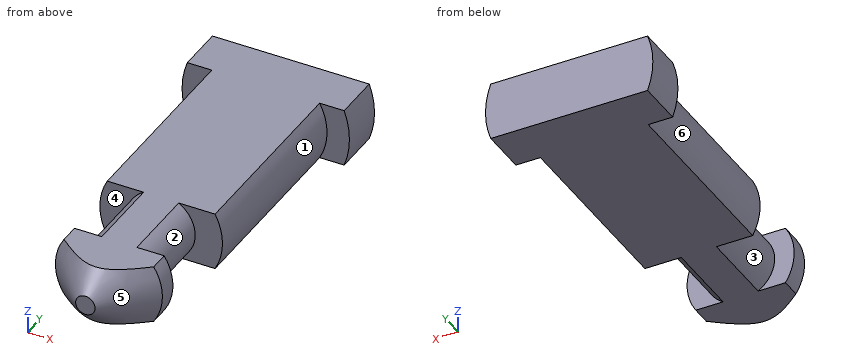
from build123d import *

# Parameters (mm, degrees)
F2_W     = 15
F2_H     = 3
F3_DEPTH = 25


with BuildPart() as f1:
    # F0 (on Top) → F1 (revolve)
    with BuildSketch(Plane.XY):
        Polygon((0, 19.65), (0, 0), (0.5, 0), (2.75, 2.25), (2.75, 3.25), (1.75, 3.25), (1.75, 7.25), (3.15, 7.25), (3.15, 17.25), (4.3, 17.25), (4.3, 19.65), align=None)
    revolve(axis=Axis((0, 9.825, 0), (0, 1, 0)))


with BuildPart() as f3:
    # F2 (on face) → F3 (new body)
    with BuildSketch(Plane(origin=(0, 19.65, 0), x_dir=(-1, 0, 0), z_dir=(0, 1, 0))):
        Rectangle(F2_W, F2_H)
    extrude(amount=-F3_DEPTH)

    # F4: intersect F1
    add(f1.part, mode=Mode.INTERSECT)


solid = f3.part
Verification items for the finished model (mm, model axes). Face numbers are marked on the shaded views. A direction names the side the tool comes from. Give positions to 0.01 mm unless a question says otherwise; leave off trailing zeros. Write each loop counter-clockwise with the first axis right and the second up, starting at its lowest first coordinate (ties: lowest second). Pieces come first, ordered by that corner, then holes. Notation, with made-up numbers: (5, 23.5) - (35, 23.5) arc R31 ccw to (35, 53.5) - close; hole circle Ø5 at (80, 70). An arc over 180 degrees is marked (long way). Answer as CSV lines item,"result". Start each with the question number.
1. Thickness scan on line 1 (Y direction, x = 3.25, z = -1.25); line 2 (Y direction, x = 2.25, z = 0.8); line 3 (Y direction, x = 2.75, z = -0.9). Record the ranges inside material, lowest first.
2. Sectioned sample at D-D (y = 11.5). Record the boundary of the cut face in (x, z).
3. Draft check along Y on the marked faces 4, 5 and 6. Enter one of: pulls with the +Y half, pulls with the -Y half, needs draft (parallel to the pull), parting line crosses it, or undercut.
4. Depth check by flat-ended pin: pin 1 (0.5 mm diameter, centred on x = 3.5, z = 0, fed in from -Y); pin 2 (0.8 mm diameter, centred on x = -3.5, z = 0, fed in from -Y); pin 3 (1.8 mm diameter, centred on x = 2.5, z = -0.5, fed in from -Y). Enter the tip coordinate at first touch or a pass-through.
5. Set-up check for the marked faces 1, 2 and 3: record each of +Z, -Z, +X, -X, +Y, -Y from which the full face is reachable in a straight line by a thin tool's end or side.
6. Sectioned sample at A-A (z = 0). Record the boundary of the cut face in (x, y).
7. Sectioned sample at B-B (x = 0). Record the boundary of the cut face in (y, z).
8. Sectioned sample at C-C (y = 6.75). Record the boundary of the cut face in (x, z), then the cut area to 3 significant figures.
Derived:
1,line 1,"17.25 to 19.65"
1,line 2,"1.89 to 3.25, 7.25 to 19.65"
1,line 3,"7.25 to 19.65"
2,outline,"(-2.77, -1.5) - (2.77, -1.5) arc R3.15 ccw to (2.77, 1.5) - (-2.77, 1.5) arc R3.15 ccw to start"
3,face 4,"undercut"
3,face 5,"pulls with the -Y half"
3,face 6,"needs draft"
4,pin 1,"y = 17.25"
4,pin 2,"y = 7.25"
4,pin 3,"y = 1.15"
5,face 1,"+X, -Y"
5,face 2,"+X"
5,face 3,"-X"
6,outline,"(-4.3, 17.25) - (-3.15, 17.25) - (-3.15, 7.25) - (-1.75, 7.25) - (-1.75, 3.25) - (-2.75, 3.25) - (-2.75, 2.25) - (-0.5, 0) - (0.5, 0) - (2.75, 2.25) - (2.75, 3.25) - (1.75, 3.25) - (1.75, 7.25) - (3.15, 7.25) - (3.15, 17.25) - (4.3, 17.25) - (4.3, 19.65) - (-4.3, 19.65) - close"
7,outline,"(0, -0.5) - (1, -1.5) - (19.65, -1.5) - (19.65, 1.5) - (1, 1.5) - (0, 0.5) - close"
8,outline,"(-0.9, -1.5) - (0.9, -1.5) arc R1.75 ccw to (0.9, 1.5) - (-0.9, 1.5) arc R1.75 ccw to start"
8,area,"9.01 mm²"
